from build123d import *

# Parameters (mm, degrees)
EXTRUDE_1_DEPTH     = 2
SKETCH_4_R          = 1.5
CUT_EXTRUDE_1_DEPTH = 2


with BuildPart() as part:
    # 草图1 → 凸台-拉伸1 (new body)
    with BuildSketch(Plane(origin=(0, 0, 0), x_dir=(1, 0, 0), z_dir=(0, 1, 0))):
        with BuildLine():
            Line((-100, 15), (100, 15))
            ThreePointArc((100, 15), (115, 0), (100, -15))
            Line((100, -15), (-100, -15))
            ThreePointArc((-100, -15), (-115, 0), (-100, 15))
        make_face()
    extrude(amount=EXTRUDE_1_DEPTH)

    # 草图4 → 切除-拉伸1 (cut)
    with BuildSketch(Plane(origin=(0, 2, 0), x_dir=(1, 0, 0), z_dir=(0, 1, 0))):
        with Locations(Location((-107, 0, 0), (0, 0, 270))):
            Circle(SKETCH_4_R)
        with Locations(Location((-93, 0, 0), (0, 0, 270))):
            Circle(SKETCH_4_R)
        with Locations(Location((107, 0, 0), (0, 0, 90))):
            Circle(SKETCH_4_R)
        with Locations(Location((93, 0, 0), (0, 0, 90))):
            Circle(SKETCH_4_R)
        with Locations(Location((0, -10, 0), (0, 0, 270))):
            Circle(SKETCH_4_R)
        with Locations(Location((20, -10, 0), (0, 0, 270))):
            Circle(SKETCH_4_R)
        with Locations(Location((40, -10, 0), (0, 0, 270))):
            Circle(SKETCH_4_R)
        with Locations(Location((-20, -10, 0), (0, 0, 270))):
            Circle(SKETCH_4_R)
        with Locations(Location((-40, -10, 0), (0, 0, 270))):
            Circle(SKETCH_4_R)
        with BuildLine():
            Line((-60, 6.25), (60, 6.25))
            ThreePointArc((60, 6.25), (66.25, 0), (60, -6.25))
            Line((60, -6.25), (-60, -6.25))
            ThreePointArc((-60, -6.25), (-66.25, 0), (-60, 6.25))
        make_face()
    extrude(amount=-CUT_EXTRUDE_1_DEPTH, mode=Mode.SUBTRACT)


solid = part.part
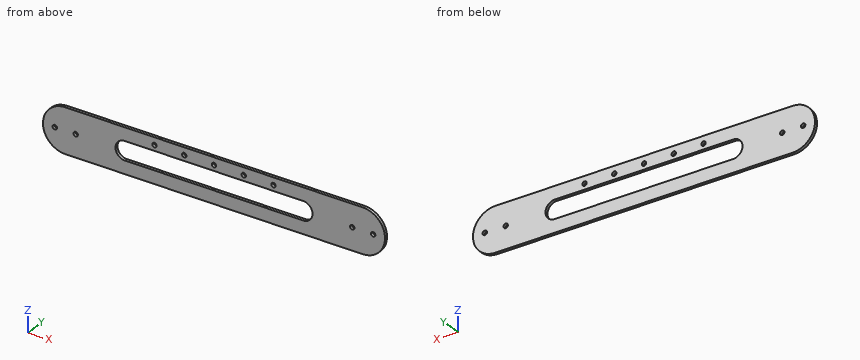
Read the model definition and answer for the solid it produces. Units are mm, in the model's axes. Coordinates: 2 decimals unless noted, no trailing zeros. Write each loop counter-clockwise with the first axis right and the second up, starting at its lowest first coordinate (ties: lowest second). Pieces come first, ordered by that corner, then holes. Notation, with made-up numbers: M 87,81.25 L 132,81.25 A23 ccw 132,109.25 Z; hole C 73.5,-32 d8. An arc over 180 degrees is marked long. Use a Markdown table: item, result.
Q1. The part is cut by section C-C, the plane z = -13. Write down the section's boundary in (x, y).
Answer block:
| item | result |
|---|---|
| outline | M -107.48,0 L 107.48,0 L 107.48,2 L -107.48,2 Z |
Q2. Straight lines are drawn through the part: L1, parallel to Z at x = -93, y = 0.5; L2, parallel to X at y = 1.4, z = 0; L3, parallel to Z at x = -9, y = 1.15. For each, find the intervals that lie inside material, in ascending order. Write a range as [from, to].
Answer block:
| item | result |
|---|---|
| L1 | z = [-15, -1.5], [1.5, 15] |
| L2 | x = [-115, -108.5], [-105.5, -94.5], [-91.5, -66.25], [66.25, 91.5], [94.5, 105.5], [108.5, 115] |
| L3 | z = [-15, -6.25], [6.25, 15] |
Q3. Each of these flat-tipped pins is pushed along its axis until it touches: pin 1 Ø4 at (x, z) = (-43.5, -10) entering from -Y; pin 2 Ø1.8 at (x, z) = (20, 10) entering from -Y. Where does it stop, or does it pass through?
Answer block:
| item | result |
|---|---|
| pin 1 | stops at y = 0 |
| pin 2 | passes through |
Q4. The part is cut by section A-A, the plane y = 1.25. Give the number of separate pieces and of enclosed holes in the cut face, then the cut area to 3 significant figures.
Answer block:
| item | result |
|---|---|
| separate pieces | 1 |
| enclosed holes | 10 |
| area | 5,020 mm2 |
Q5. The part is cut by section B-B, the plane z = -4. Write down the section's boundary in (x, y), then the cut area to 3 significant figures.
Answer block:
| item | result |
|---|---|
| outline | M -114.46,0 L -64.8,0 L -64.8,2 L -114.46,2 Z; M 64.8,0 L 114.46,0 L 114.46,2 L 64.8,2 Z |
| area | 199 mm2 |
